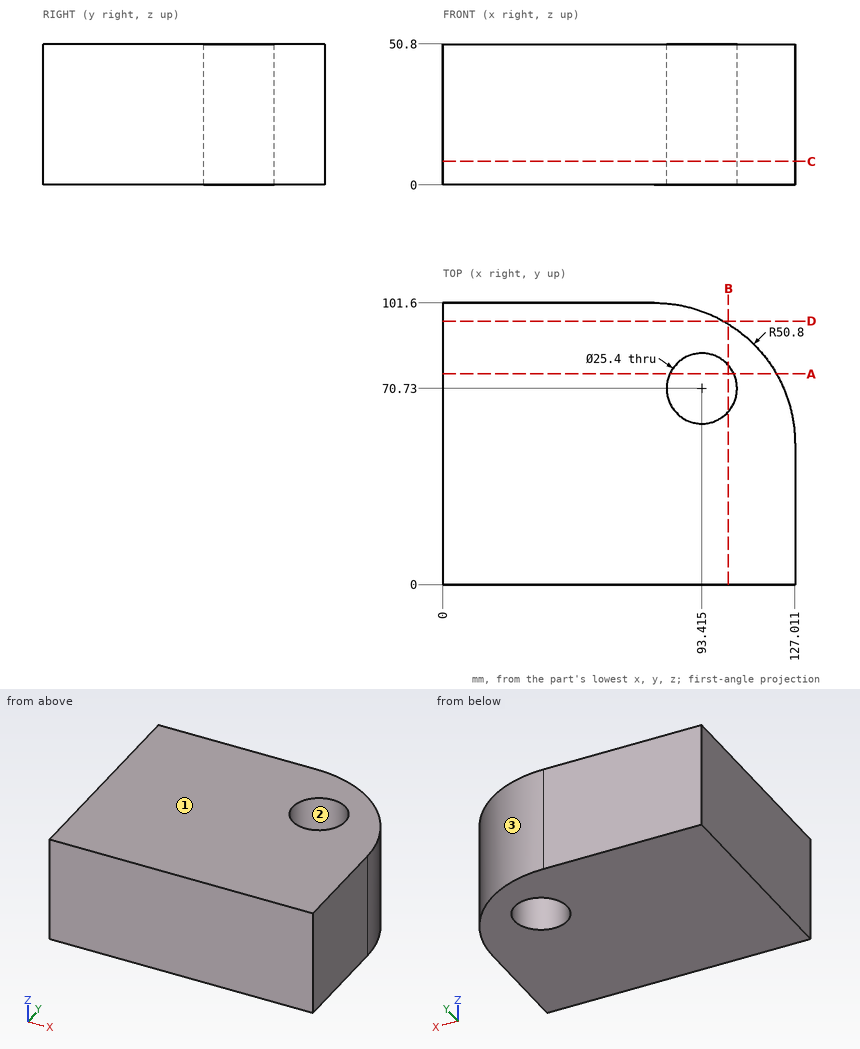
Study the drawing (mm; zero at the part's minimum x, y, z) and answer. Give positions to 0.01 mm unless a question says otherwise; leave off trailing zeros. Write each loop counter-clockwise with the first axis right and the second up, starting at its lowest first coordinate (ties: lowest second). Pieces come first, ordered by that corner, then holes.
Item 1: A flat-ended cylindrical pin translates along its axis: P1, Ø8, axis at y = 72, z = 44.5, coming from the +X side. Find the tip coordinate at first contact, or state that the pin passes through.
Item 2: Find the intervals of material crossed by line 1 along X through (y, z) = (81, 5.5) (1 decimal); line 2 along Y through (x, z) = (98.5, 30.5); line 3 along Y through (x, z) = (90, 48), in increasing order.
Item 3: Section D-D, the plane y = 95 is taken. Write down the section's boundary in (x, z), plus the area to 3 significant figures.
Item 4: Section B-B, the plane x = 103 is taken. Write down the section's boundary in (y, z).
Item 5: Section C-C, the plane z = 8.5 is taken. Write down the section's boundary in (x, y) (1 decimal).
Item 6: Determine the mould class of the marked faces 1, 2 and 3 for opening direction X: released by +X, released by -X, zero draft, split by the parting line, or undercut.
Item 7: Section A-A, the plane y = 76 is taken. Write down the section's boundary in (x, z).
Completed:
1. P1: stops at x = 124.01
2. line 1: x = 0 to 85.9, 100.9 to 117.1
2. line 2: y = 0 to 59.09, 82.37 to 96.45
2. line 3: y = 0 to 58.5, 82.96 to 99.69
3. outline: (0, 0) - (101.25, 0) - (101.25, 50.8) - (0, 50.8) - close
3. area: 5,140 mm2
4. outline: (0, 0) - (62.4, 0) - (62.4, 50.8) - (0, 50.8) - close; (79.06, 0) - (93.96, 0) - (93.96, 50.8) - (79.06, 50.8) - close
5. outline: (0, 0) - (127, 0) - (127, 50.8) arc R50.8 ccw to (76.2, 101.6) - (0, 101.6) - close; hole circle Ø25.4 at (93.4, 70.7)
6. face 1: zero draft
6. face 2: undercut
6. face 3: released by +X
7. outline: (0, 0) - (81.86, 0) - (81.86, 50.8) - (0, 50.8) - close; (104.97, 0) - (120.32, 0) - (120.32, 50.8) - (104.97, 50.8) - close
